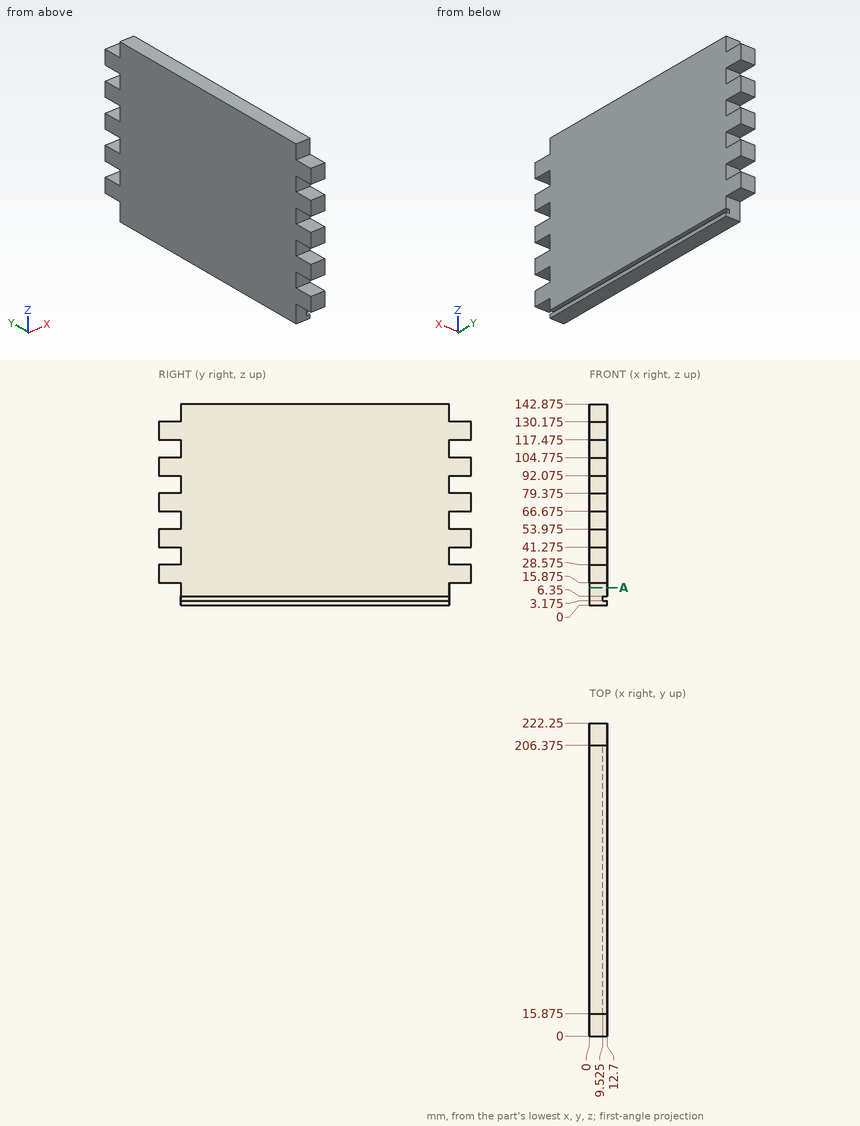
Geometry: see drawing. Coordinates: mm, zero at the bounding-box minimum. Give positions to 0.01 mm unless a question says otherwise; leave off trailing zeros. Order: outer loops, then holes, each group sorted by start corner. A loop starts at its lowest first (then second) coordinate and runs counter-clockwise, first axis right, second up. Notation, with made-up numbers: (83, -18.5) -> (100, -18.5) arc R26 ccw to (100, 15.5) -> close; hole circle Ø2 at (35.5, 29). An arc over 180 degrees is marked (long way). Write each question's results on one line, items separated by ' | '. Start each with the question number.
1) Section A-A (z = 12.5). Return loops of the section in (x, y) (3 decimals), then the cut area to 3 significant figures.
2) Line query: line 1 (Z direction, x = 12.25, y = 169) (3 decimals); line 2 (Y direction, x = 7.5, z = 106) (3 decimals). Output: solid intervals per line, ascending. Write a range as from..to.
3) First-contact query: pin 1 (6.5 mm diameter, centred on x = 7, y = 213, fed in from -Z) (3 decimals); pin 2 (4 mm diameter, centred on x = 7.5, z = 87, fed in from -Y) (3 decimals); pin 3 (6.5 mm diameter, centred on x = 5, z = 109, fed in from +Y) (3 decimals). Flat tips, straight axial feed; report the tip coordinate or a pass-through.
Calculated:
1) outline: (0, 15.875) -> (12.7, 15.875) -> (12.7, 206.375) -> (0, 206.375) -> close | area: 2,420 mm2
2) line 1: 0..3.175, 6.35..142.875 | line 2: 15.875..206.375
3) pin 1: z = 15.875 | pin 2: y = 15.875 | pin 3: y = 206.375
